Autodesk Inventor part; units mm, degrees
ref_plane "YZ Plane" through (0, 0, 0) normal (1, 0, 0) x (0, 1, 0)
ref_plane "XZ Plane" through (0, 0, 0) normal (0, 1, 0) x (-1, 0, 0)
ref_plane "XY Plane" through (0, 0, 0) normal (0, 0, 1) x (1, 0, 0)
sketch "Sketch1" plane through (0, 0, 0) normal (1, 0, 0) x (0, 1, 0)
  arc A0 (-3.4641, 2) -> (3.4641, 2) centre (0, 0) ccw
  arc A1 (-5.1962, 3) -> (5.1962, 3) centre (0, 0) ccw
  arc A2 (5.1962, 3) -> (3.4641, 2) centre (4.3301, 2.5) ccw
  arc A3 (-3.4641, 2) -> (-5.1962, 3) centre (-4.3301, 2.5) ccw
  dimension "d0" = 8
  dimension "d1" = 12
  dimension "d2" = 2.5
extrude "Extrusion1" add sketch "Sketch1" against normal blind 26
sketch "Sketch2" plane through (0, 0, 0) normal (1, 0, 0) x (0, 0, -1)
  line L0 (-7.4, 15) -> (3.6, 15)
  line L1 (3.6, 15) -> (3.6, 4)
  line L2 (3.6, 4) -> (-7.4, 4)
  line L3 (-7.4, 4) -> (-7.4, 15)
  arc A0 (-2, -3.4641) -> (-2, 3.4641) centre (0, 0) ccw
  line L4 (-7.4, 15) -> (-1.9, 15)
  line L5 (-1.9, 15) -> (-1.9, 8)
  line L6 (-1.9, 8) -> (-7.4, 8)
  line L7 (-7.4, 8) -> (-7.4, 15)
  dimension "d5" = 11
  dimension "d6" = 11
  dimension "d7" = 7.4
  dimension "d8" = 5.5
  dimension "d9" = 7
extrude "Extrusion2" add sketch "Sketch2" along normal blind 3 contours L0 L5 L6 L3
sketch "Sketch3" plane through (0, 0, 0) normal (-1, 0, 0) x (0, 0, 1)
  line L0 (7.4, 15) -> (7.4, 8)
  line L1 (7.4, 15) -> (-1.9, 15)
  line L2 (1.9, 8) -> (7.4, 8)
  line L3 (7.4, 8) -> (7.4, 15)
  arc A0 (2, 3.4641) -> (2, -3.4641) centre (0, 0) ccw
  line L4 (7.4, 8) -> (1.9, 8)
  line L5 (1.9, 8) -> (1.9, 15)
  line L6 (1.9, 8) -> (1.9, 5.6912)
  arc A1 (3, 5.1962) -> (3, -5.1962) centre (0, 0) ccw
  line L7 (-1.9, 15) -> (-1.9, 5.6912)
  dimension "d12" = 1.9
extrude "Extrusion3" add sketch "Sketch3" along normal blind 3
fillet "Fillet1" radius 2 3 edges at (-1.5, 5.6912, 1.9) (-1.5, 5.6912, -1.9) (-1.5, 15, -1.9)
sketch "Sketch4" plane through (-26, 0, 0) normal (-1, 0, 0) x (0, 0, 1)
  line L0 (7.6885, 0) -> (-10.3871, 0)
  line L1 (-10.3871, 0) -> (-10.3871, 6.8992)
  line L2 (-10.3871, 6.8992) -> (7.6885, 6.8992)
  line L3 (7.6885, 6.8992) -> (7.6885, 0)
  point P0 (0, 0)
extrude "Extrusion4" cut sketch "Sketch4" against normal blind 3
properties part number "Roller_Spacer_P"
Input: part model. Units: mm. Frame: model coordinates. A direction names the side the tool comes from. Round coordinates to 2 decimals unless told otherwise and drop trailing zeros. Loops run counter-clockwise (first coordinate to the right, second up) from the corner with the lowest first, then second, coordinate; pieces in that order, holes last. Notation, with made-up numbers: M 79,-24 L 117,-24 A24 cw 117,-2 Z; hole C 88,55.5 d6. An arc over 180 degrees is marked long. Answer in a Markdown table with one row per item. Add a question column.
1. Ray query, probe 1 along Y at (x, z) = (-11.5, 0); probe 2 along Z at (x, y) = (-19.5, 0); probe 3 along X at (y, z) = (2.25, -4.75). Return the intervals inside material, ascending.
2. Section B-B (x = -0.5). Output: boundary loops of the cut face in (y, z) (3 decimals), and give its area (3 significant figures).
3. Set-up query: faces 1 (the face through (-1, 10, -1.9)), 2 (the face through (-23, 4, -2)), 3 (the face through (1, 12, 1.9)). Return all of +Z, -Z, +X, -X, +Y, -Y with unobstructed straight access to the full face (end or side cutting, diameter ignored); none if empty.
4. Section D-D (y = -1.75). Output: boundary loops of the cut face in (x, z).
5. Contact query for flat-ended pins moving along their axis: pin 1 (3 mm diameter, centred on y = 12, z = 1.5, fed in from -X); pin 2 (3.5 mm diameter, centred on x = -1, y = 10, fed in from -Z); pin 3 (12 mm diameter, centred on x = -0.5, y = 7.5, fed in from +Z); pin 4 (1 mm diameter, centred on x = -25, z = -5.5, fed in from +Y). Output: stop coordinate, or through.
6. Mould query, pull axis Y, two halves, no side actions, for faces 4 (the face through (-1.521, 5.96, -2.183)), 5 (the face through (3, 12, 5)), 6 (the face through (-12.818, -3.811, 3.355)). Classes: released by +Y, released by -Y, zero draft, split by the parting line, or undercut.
7. Section C-C (z = -2.25). Output: boundary loops of the cut face in (x, y).
8. Section A-A (z = 1). Output: boundary loops of the cut face in (x, y).
Values follow:
| question | item | result |
|---|---|---|
| 1 | probe 1 | -6 to -4, 4 to 6 |
| 1 | probe 2 | -6 to -4 |
| 1 | probe 3 | -23 to 0 |
| 2 | outline | M -5.196,3 A6 ccw long 5.239,-2.925 A2 cw 6.985,-1.9 L 13,-1.9 A2 ccw 15,0.1 L 15,7.4 L 8,7.4 L 8,1.9 L 6.985,1.9 A2 cw 5.239,2.925 A6 ccw 5.196,3 A1 ccw 3.464,2 A4 cw long -3.464,2 A1 ccw Z |
| 2 | area | 118 mm^2 |
| 3 | face 1 | -Z, +X, -X, +Y |
| 3 | face 2 | +Z, -Z, -X, +Y |
| 3 | face 3 | -Z, +X, +Y, -Y |
| 4 | outline | M -26,-5.74 L 0,-5.74 L 0,-3.6 L -26,-3.6 Z |
| 5 | pin 1 | x = -3 |
| 5 | pin 2 | z = -1.9 |
| 5 | pin 3 | z = 7.4 |
| 5 | pin 4 | y = 0 |
| 6 | face 4 | released by +Y |
| 6 | face 5 | zero draft |
| 6 | face 6 | undercut |
| 7 | outline | M -26,-5.56 L 0,-5.56 L 0,-3.31 L -26,-3.31 Z; M -23,3.31 L 0,3.31 L 0,5.85 L -3,5.85 L -3,5.56 L -23,5.56 Z |
| 8 | outline | M -26,-5.92 L 0,-5.92 L 0,-3.87 L -26,-3.87 Z; M -23,3.87 L 0,3.87 L 0,15 L -3,15 L -3,5.92 L -23,5.92 Z |
